Design review of the part shown in the three views and the two pictorial views. Dimensions are in mm from the part's minimum x, y and z. A direction names the side the tool comes from. Round coordinates to 2 decimals unless told otherwise and drop trailing zeros. Write each loop counter-clockwise with the first axis right and the second up, starting at its lowest first coordinate (ties: lowest second). Pieces come first, ordered by that corner, then holes. Notation, with made-up numbers: (0, 27) - (58, 27) arc R4 ccw to (58, 33) - close; hole circle Ø4 at (66.25, 74.25). An arc over 180 degrees is marked (long way). Use one line per item in the form item = value.
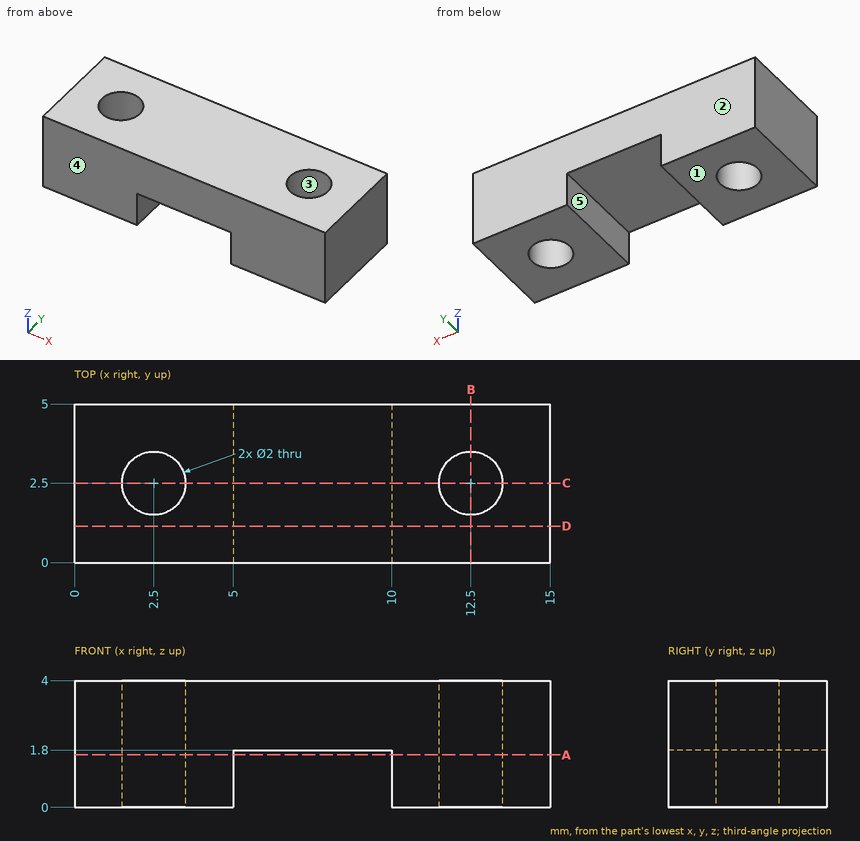
Q1. We need section B-B on x = 12.5. Write out the cut boundary in (y, z).
Calculated:
outline = (0, 0) - (1.5, 0) - (1.5, 4) - (0, 4) - close; (3.5, 0) - (5, 0) - (5, 4) - (3.5, 4) - close
Q2. For P1, Ø1.6, axis at x = 2.5, y = 2.5, coming from the -Z side, flat-tipped, find the tip position at first contact; note if it passes through.
Calculated:
P1 = through
Q3. We need section C-C on y = 2.5. Write out the cut boundary in (x, z), then the cut area to 3 significant figures.
Calculated:
outline = (0, 0) - (1.5, 0) - (1.5, 4) - (0, 4) - close; (3.5, 0) - (5, 0) - (5, 1.8) - (10, 1.8) - (10, 0) - (11.5, 0) - (11.5, 4) - (3.5, 4) - close; (13.5, 0) - (15, 0) - (15, 4) - (13.5, 4) - close
area = 35.0 mm2
Q4. Machinability: for the marked faces 4 and 5, which of the approach directions +Z, -Z, +X, -X, +Y, -Y give a long, thin tool a straight path to every point of the face, cutting with its end or side? Answer none if there is none.
Calculated:
face_4 = +Z, -Z, +X, -X, -Y
face_5 = -Z, +Y, -Y
Q5. Draft analysis for pull direction Y (two halves, no side actions). For the marked faces 1, 2 and 3, state which applies: released by +Y, released by -Y, zero draft, split by the parting line, or undercut.
Calculated:
face_1 = zero draft
face_2 = released by +Y
face_3 = undercut
Q6. We need section A-A on z = 1.65. Write out the cut boundary in (x, y), then the cut area to 3 significant figures.
Calculated:
outline = (0, 0) - (5, 0) - (5, 5) - (0, 5) - close; (10, 0) - (15, 0) - (15, 5) - (10, 5) - close; hole circle Ø2 at (2.5, 2.5); hole circle Ø2 at (12.5, 2.5)
area = 43.7 mm2
Q7. To check wall thickness, follow line 1 along Y through (x, z) = (2.5, 1.7); line 2 along X through (y, z) = (2.85, 2.2); line 3 along Z through (x, y) = (8.5, 4.7). State the ranges of each line that lie inside material, in increasing order. Write a range as from..to.
Calculated:
line_1 = 0..1.5, 3.5..5
line_2 = 0..1.56, 3.44..11.56, 13.44..15
line_3 = 1.8..4
Q8. We need section D-D on y = 1.15. Write out the cut boundary in (x, z), then the cut area to 3 significant figures.
Calculated:
outline = (0, 0) - (5, 0) - (5, 1.8) - (10, 1.8) - (10, 0) - (15, 0) - (15, 4) - (0, 4) - close
area = 51.0 mm2
